```python
from build123d import *

# Parameters (mm, degrees)
SKETCH8_W                                        = 65.5
SKETCH8_H                                        = 65.7
BOSS_EXTRUDE6_DEPTH                              = 4
SKETCH8_3_R                                      = 4.25
BOSS_EXTRUDE7_DEPTH                              = 35.5
SKETCH8_3_W                                      = 33.85
SKETCH8_3_H                                      = 43.5
BOSS_EXTRUDE7_2_DEPTH                            = 35.5
SKETCH8_4_W                                      = 45
SKETCH8_4_H                                      = 43.5
SKETCH8_4_R                                      = 11.8
BOSS_EXTRUDE8_DEPTH                              = 10
BOSS_EXTRUDE9_DEPTH                              = 62
SKETCH8_6_W                                      = 20
SKETCH8_6_H                                      = 4
BOSS_EXTRUDE10_DEPTH                             = 35.5
CBORE_FOR_M3_PAN_HEAD_MACHINE_SCREW2_D           = 3.4
CBORE_FOR_M3_PAN_HEAD_MACHINE_SCREW2_CBORE_D     = 7
CBORE_FOR_M3_PAN_HEAD_MACHINE_SCREW2_CBORE_DEPTH = 2.4
SKETCH13_R                                       = 4.75
CUT_EXTRUDE1_DEPTH                               = 2
CBORE_FOR_M4_PAN_HEAD_MACHINE_SCREW1_D           = 4.5
CBORE_FOR_M4_PAN_HEAD_MACHINE_SCREW1_CBORE_D     = 9
CBORE_FOR_M4_PAN_HEAD_MACHINE_SCREW1_CBORE_DEPTH = 3.1
SKETCH14_W                                       = 65.5
SKETCH14_H                                       = 65.7
BOSS_EXTRUDE11_DEPTH                             = 28.4
CUT_EXTRUDE2_REACH                               = 170.332
SKETCH17_R                                       = 11.6
CUT_EXTRUDE3_REACH                               = 158.114
SKETCH19_R                                       = 5.25
CBORE_START                                      = -14.812673424
CBORE_FOR_M3_PAN_HEAD_MACHINE_SCREW3_OUT_R       = 1.6
CBORE_FOR_M3_PAN_HEAD_MACHINE_SCREW3_DEPTH       = 14.812673424
CBORE_START_2                                    = -2.4
CBORE_FOR_M3_PAN_HEAD_MACHINE_SCREW3_2_O_R       = 3.5
CBORE_FOR_M3_PAN_HEAD_MACHINE_SCREW3_2_O_R_2     = 1.6
CBORE_FOR_M3_PAN_HEAD_MACHINE_SCREW3_2_DEPTH     = 2.4


# Read off the part's stored shape, not the designer's step: CBORE for M3 Pan Head Machine Screw3
with BuildPart() as part:
    # Sketch8 → Boss-Extrude6 (new body)
    with BuildSketch(Plane.XY):
        with Locations((0, -79.35)):
            Rectangle(SKETCH8_W, SKETCH8_H)
    extrude(amount=-BOSS_EXTRUDE6_DEPTH)



with BuildPart() as body_2:
    # Sketch8<3> → Boss-Extrude7 (new body)
    with BuildSketch(Plane.XY):
        Polygon((-22.5, 0), (-56.35, 0), (-56.35, -4), (-56.35, -43.5), (-22.5, -43.5), align=None)
        with Locations((-40, -18.75)):
            Circle(SKETCH8_3_R, mode=Mode.SUBTRACT)
    extrude(amount=-BOSS_EXTRUDE7_DEPTH)



with BuildPart() as body_3:
    # Sketch8<3> → Boss-Extrude7 2 (new body)
    with BuildSketch(Plane.XY):
        with Locations((39.425, -21.75)):
            Rectangle(SKETCH8_3_W, SKETCH8_3_H)
        with Locations((40, -18.75)):
            Circle(SKETCH8_3_R, mode=Mode.SUBTRACT)
    extrude(amount=-BOSS_EXTRUDE7_2_DEPTH)


with BuildPart() as body_2_1:
    add(body_2.part)

    add(body_3.part)  # Boss-Extrude8 merges body 3
    # Sketch8<4> → Boss-Extrude8 (add)
    with BuildSketch(Plane.XY):
        with Locations((0, -21.75)):
            Rectangle(SKETCH8_4_W, SKETCH8_4_H)
        with Locations((0, -21.75)):
            Circle(SKETCH8_4_R, mode=Mode.SUBTRACT)
    extrude(amount=-BOSS_EXTRUDE8_DEPTH)


with BuildPart() as part_1:
    add(part.part)

    add(body_2_1.part)  # Boss-Extrude9 merges body 2
    # Sketch8<5> → Boss-Extrude9 (add)
    with BuildSketch(Plane.XY):
        Polygon((22.5, -43.5), (-22.5, -43.5), (-56.35, -43.5), (-56.35, -46.5), (-32.75, -46.5), (32.75, -46.5), (56.35, -46.5), (56.35, -43.5), align=None)
    extrude(amount=-BOSS_EXTRUDE9_DEPTH)

    # Sketch8<6> → Boss-Extrude10 (add)
    with BuildSketch(Plane.XY):
        with Locations((-66.35, -2)):
            Rectangle(SKETCH8_6_W, SKETCH8_6_H)
    extrude(amount=-BOSS_EXTRUDE10_DEPTH)

    # CBORE for M3 Pan Head Machine Screw2 (through all)
    with Locations(Plane(origin=(-15.5, -6.25, 0), x_dir=(1, 0, 0), z_dir=(0, 0, 1))):
        with Locations((0, 0), (31, 0), (31, -31), (0, -31)):
            CounterBoreHole(CBORE_FOR_M3_PAN_HEAD_MACHINE_SCREW2_D / 2, CBORE_FOR_M3_PAN_HEAD_MACHINE_SCREW2_CBORE_D / 2, CBORE_FOR_M3_PAN_HEAD_MACHINE_SCREW2_CBORE_DEPTH)

    # Sketch13 → Cut-Extrude1 (cut)
    with BuildSketch(Plane.XY):
        with Locations((-20, -59.6)):
            Circle(SKETCH13_R)
        with Locations((20, -99.3)):
            Circle(SKETCH13_R)
        with Locations((-20, -99.3)):
            Circle(SKETCH13_R)
        with Locations((20, -59.6)):
            Circle(SKETCH13_R)
    extrude(amount=-CUT_EXTRUDE1_DEPTH, mode=Mode.SUBTRACT)

    # CBORE for M4 Pan Head Machine Screw1 (through all)
    with Locations(Plane(origin=(10, -59.6, -4), x_dir=(-1, 0, 0), z_dir=(0, 0, -1))):
        with Locations((0, 0), (20, 0), (0, -39.7), (20, -39.7)):
            CounterBoreHole(CBORE_FOR_M4_PAN_HEAD_MACHINE_SCREW1_D / 2, CBORE_FOR_M4_PAN_HEAD_MACHINE_SCREW1_CBORE_D / 2, CBORE_FOR_M4_PAN_HEAD_MACHINE_SCREW1_CBORE_DEPTH)

    # Sketch14 → Boss-Extrude11 (add)
    with BuildSketch(Plane(origin=(0, 0, -4), x_dir=(-1, 0, 0), z_dir=(0, 0, -1))):
        with Locations((0, -79.35)):
            Rectangle(SKETCH14_W, SKETCH14_H)
        with BuildLine():
            Line((15.25, -61.65), (15.25, -97.25))
            Line((15.25, -97.25), (14.560427612, -97.25))
            ThreePointArc((14.560427612, -97.25), (14.888871959, -98.251700915), (15, -99.3))
            ThreePointArc((15, -99.3), (8.951700915, -104.188871959), (5.439572388, -97.25))
            Line((5.439572388, -97.25), (-5.439572388, -97.25))
            ThreePointArc((-5.439572388, -97.25), (-5.111128041, -98.251700915), (-5, -99.3))
            ThreePointArc((-5, -99.3), (-11.048299085, -104.188871959), (-14.560427612, -97.25))
            Line((-14.560427612, -97.25), (-15.25, -97.25))
            Line((-15.25, -97.25), (-15.25, -61.65))
            Line((-15.25, -61.65), (-14.560427612, -61.65))
            ThreePointArc((-14.560427612, -61.65), (-11.048299085, -54.711128041), (-5, -59.6))
            ThreePointArc((-5, -59.6), (-5.111128041, -60.648299085), (-5.439572388, -61.65))
            Line((-5.439572388, -61.65), (5.439572388, -61.65))
            ThreePointArc((5.439572388, -61.65), (8.951700915, -54.711128041), (15, -59.6))
            ThreePointArc((15, -59.6), (14.888871959, -60.648299085), (14.560427612, -61.65))
            Line((14.560427612, -61.65), (15.25, -61.65))
        make_face(mode=Mode.SUBTRACT)
    extrude(amount=BOSS_EXTRUDE11_DEPTH)

    # Sketch17 → Cut-Extrude2 (cut, up to next)
    with BuildSketch(Plane(origin=(32.75, 0, 0), x_dir=(0, 0, -1), z_dir=(1, 0, 0)), mode=Mode.PRIVATE) as cut_extrude2_sk1:
        with Locations(Location((19.1, -79.45, 0), (0, 0, 90))):
            Circle(SKETCH17_R)
    cut_extrude2_tool1 = extrude(cut_extrude2_sk1.sketch, amount=-CUT_EXTRUDE2_REACH, mode=Mode.PRIVATE) & part_1.part
    add(cut_extrude2_tool1.solids().sort_by_distance((32.75, -79.45, -19.1))[0], mode=Mode.SUBTRACT)

    # Sketch19 → Cut-Extrude3 (cut, up to next)
    with BuildSketch(Plane.ZY.offset(32.75), mode=Mode.PRIVATE) as cut_extrude3_sk1:
        with Locations(Location((-19.1, -79.45, 0), (0, 0, 270))):
            Circle(SKETCH19_R)
    cut_extrude3_tool1 = extrude(cut_extrude3_sk1.sketch, amount=-CUT_EXTRUDE3_REACH, mode=Mode.PRIVATE) & part_1.part
    add(cut_extrude3_tool1.solids().sort_by_distance((-32.75, -79.45, -19.1))[0], mode=Mode.SUBTRACT)

    # CBORE for M3 Pan Head Machine Screw3 out → CBORE for M3 Pan Head Machine Screw3 (cut)
    with BuildSketch(Plane(origin=(0, 0, 0), x_dir=(1, 0, 0), z_dir=(0, 1, 0)).offset(CBORE_START)):
        with Locations((-40, 17.75)):
            Circle(CBORE_FOR_M3_PAN_HEAD_MACHINE_SCREW3_OUT_R)
        with Locations((40, 17.75)):
            Circle(CBORE_FOR_M3_PAN_HEAD_MACHINE_SCREW3_OUT_R)
    extrude(amount=CBORE_FOR_M3_PAN_HEAD_MACHINE_SCREW3_DEPTH, mode=Mode.SUBTRACT)

    # CBORE for M3 Pan Head Machine Screw3 2 o → CBORE for M3 Pan Head Machine Screw3 2 (cut)
    # profile 1 of 2: a face of its own
    with BuildSketch(Plane(origin=(0, 0, 0), x_dir=(1, 0, 0), z_dir=(0, 1, 0)).offset(CBORE_START_2)):
        with Locations((-40, 17.75)):
            Circle(CBORE_FOR_M3_PAN_HEAD_MACHINE_SCREW3_2_O_R)
        with Locations((-40, 17.75)):
            Circle(CBORE_FOR_M3_PAN_HEAD_MACHINE_SCREW3_2_O_R_2, mode=Mode.SUBTRACT)
    # profile 2 of 2: a face of its own
    with BuildSketch(Plane(origin=(0, 0, 0), x_dir=(1, 0, 0), z_dir=(0, 1, 0)).offset(CBORE_START_2)):
        with Locations((40, 17.75)):
            Circle(CBORE_FOR_M3_PAN_HEAD_MACHINE_SCREW3_2_O_R)
        with Locations((40, 17.75)):
            Circle(CBORE_FOR_M3_PAN_HEAD_MACHINE_SCREW3_2_O_R_2, mode=Mode.SUBTRACT)
    extrude(amount=CBORE_FOR_M3_PAN_HEAD_MACHINE_SCREW3_2_DEPTH, mode=Mode.SUBTRACT)


solid = part_1.part
```
Here's how the part is built. I have some questions about the finished solid (model axes, mm). A direction names the side the tool comes from. Coordinates: 2 decimals unless noted, no trailing zeros. Order: outer loops, then holes, each group sorted by start corner. A loop starts at its lowest first (then second) coordinate and runs counter-clockwise, first axis right, second up. Notation, with made-up numbers: (74, 66.25) -> (120, 66.25) arc R11 ccw to (120, 81.25) -> close; hole circle Ø10 at (24, 60). An arc over 180 degrees is marked (long way). Return JSON: item names as keys, results as strings.
1) On a 3-axis mill with a long thin cutter (end or side, diameter ignored), from which of +Z, -Z, +X, -X, +Y, -Y can I reach the whole of each face in a straight line? I mean faces 5 (the flat face through (0, -97.25, -18)), 6 (the flat face through (-32.75, -80, -12)), 7 (the flat face through (-14, -36, -2.4)), 8 (the flat face through (-1, -46.5, -37)), 9 (the flat face through (-10, -31, -10)). Say none if no direction works.
Conclusion:
{"face 5": "-Z", "face 6": "+Z, -Z, -X, -Y", "face 7": "+Z", "face 8": "-Z, -Y", "face 9": "-Z, +Y"}
2) Thinking about a two-plate mould opening in X: for faces 1 (the cylindrical face through (-10.29, -97.07, -0.44)), 2 (the cylindrical face through (24.123, -68.735, -23.543)), 3 (the flat face through (56.35, -24, -17)), 4 (the flat face through (15.25, -92, -18)), which applies, +X half, -X half, draft (parallel to the pull), parting line (faces both ways), or undercut?
Conclusion:
{"face 1": "undercut", "face 2": "draft", "face 3": "+X half", "face 4": "undercut"}
3) If we section it at D-D on x = 0.5: List the corners of the cut face in (y, z) for me.
Conclusion:
{"outline": "(-112.2, -32.4) -> (-97.25, -32.4) -> (-97.25, -4) -> (-61.65, -4) -> (-61.65, -32.4) -> (-46.5, -32.4) -> (-46.5, -62) -> (-43.5, -62) -> (-43.5, -10) -> (-33.54, -10) -> (-33.54, 0) -> (-112.2, 0) -> close; (-9.96, -10) -> (0, -10) -> (0, 0) -> (-9.96, 0) -> close"}
4) If I drill on probe 1 along Y at (x, z) = (-10, -2.95); probe 2 along Y at (x, z) = (4.5, -11); probe 3 along X at (y, z) = (-8.5, -17.75), over which ranges is the centre line in solid material (lowest first)?
Conclusion:
{"probe 1": "y = -112.2 to -103.8, -94.8 to -64.1, -55.1 to -28.01, -15.49 to 0", "probe 2": "y = -112.2 to -97.25, -61.65 to -43.5", "probe 3": "x = -56.35 to -41.6, -38.4 to -22.5, 22.5 to 38.4, 41.6 to 56.35"}
5) If we section it at B-B on y = -79.45: List the corners of the cut face in (x, z) for me, plus the area to 3 significant figures.
Conclusion:
{"outline": "(-32.75, -32.4) -> (-15.25, -32.4) -> (-15.25, -24.35) -> (-32.75, -24.35) -> close; (-32.75, -13.85) -> (-15.25, -13.85) -> (-15.25, -4) -> (15.25, -4) -> (15.25, -7.5) -> (32.75, -7.5) -> (32.75, 0) -> (-32.75, 0) -> close; (15.25, -32.4) -> (32.75, -32.4) -> (32.75, -30.7) -> (15.25, -30.7) -> close", "area": "666 mm²"}
6) If we section it at A-A on y = -6.25: List the corners of the cut face in (x, z) for me, plus the area to 3 significant figures.
Conclusion:
{"outline": "(-56.35, -35.5) -> (-22.5, -35.5) -> (-22.5, -10) -> (-17.2, -10) -> (-17.2, -2.4) -> (-19, -2.4) -> (-19, 0) -> (-56.35, 0) -> close; (-13.8, -10) -> (13.8, -10) -> (13.8, -2.4) -> (12, -2.4) -> (12, 0) -> (-12, 0) -> (-12, -2.4) -> (-13.8, -2.4) -> close; (17.2, -10) -> (22.5, -10) -> (22.5, -35.5) -> (56.35, -35.5) -> (56.35, 0) -> (19, 0) -> (19, -2.4) -> (17.2, -2.4) -> close; hole circle Ø3.2 at (-40, -17.75); hole circle Ø3.2 at (40, -17.75)", "area": "2,750 mm²"}
7) If we section it at C-C on z = -6: State how many separate pieces and enclosed holes the cut face has, plus the area to 3 significant figures.
Conclusion:
{"separate pieces": "1", "enclosed holes": "8", "area": "7,710 mm²"}
8) I'm going to push flat-ended pins straight in: P1, Ø8, axis at x = -21, z = -10.5, coming from the +Y side; P2, Ø1.5, axis at x = 14, z = -52, coming from the -Y side; P3, Ø4, axis at x = 15.5, y = -6.25, coming from the -Z side; P4, Ø5, axis at y = -53, z = -30.5, coming from the -X side. Where does each tip first touch, or does it pass through?
Conclusion:
{"P1": "stops at y = 0", "P2": "stops at y = -46.5", "P3": "stops at z = -10", "P4": "stops at x = -32.75"}
